Design review of the part built by this model. Coordinates are the model's own, in mm. Face numbers are marked on the shaded views. A direction names the side the tool comes from. Round coordinates to 2 decimals unless told otherwise and drop trailing zeros. Order: outer loops, then holes, each group sorted by start corner. A loop starts at its lowest first (then second) coordinate and runs counter-clockwise, first axis right, second up. Notation, with made-up numbers: (57.5, 14.25) - (84.5, 14.25) arc R29 ccw to (84.5, 45.25) - close; hole circle Ø3 at (15.5, -11). An arc over 180 degrees is marked (long way). Write item = value, one per line.
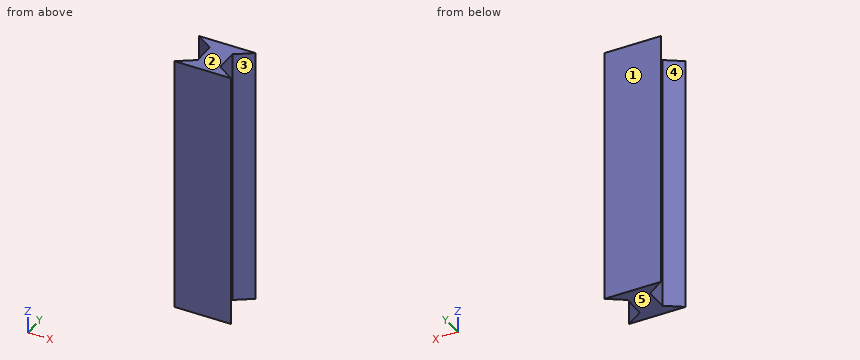
Autodesk Fusion 360 part; units mm, degrees
sketch "Sketch1" plane through (0, 0, 0) normal (0, 0, 1) x (1, 0, 0)
  line L0 (125, 0) -> (125, 1)
  line L1 (127, 0) -> (127, 1)
  line L2 (125, 0) -> (127, 0)
  line L3 (126, 0) -> (126, 2) construction
  line L4 (123.5, 2) -> (128.5, 2)
  line L5 (123.5, 2) -> (125, 1)
  line L6 (127, 1) -> (128.5, 2)
  line L7 (125, 0) -> (125, -1)
  line L8 (123.5, -2) -> (125, -1)
  line L9 (123.5, -2) -> (128.5, -2)
  line L10 (127, -1) -> (128.5, -2)
  line L11 (127, 0) -> (127, -1)
  line L12 (125, 0) -> (127, 0)
  dimension "d759" = 1
  dimension "d760" = 1
  dimension "d761" = 2
  dimension "d763" = 2
  dimension "d764" = 5
extrude "Extrude1" add sketch "Sketch1" along normal blind 23
Item 1: Take a section at D-D, the plane y = -1.2. State the section outline as (x, z) points, and give its area (3 significant figures).
Data:
outline = (124.7, 0) - (127.3, 0) - (127.3, 23) - (124.7, 23) - close
area = 59.8 mm2
Item 2: Take a section at C-C, the plane y = 0.45. State the section outline as (x, z) points, and give its area (3 significant figures).
Data:
outline = (125, 0) - (127, 0) - (127, 23) - (125, 23) - close
area = 46.0 mm2
Item 3: Take a section at B-B, the plane x = 124.75. State the section outline as (y, z) points.
Data:
outline = (-2, 0) - (-1.17, 0) - (-1.17, 23) - (-2, 23) - close; (1.17, 0) - (2, 0) - (2, 23) - (1.17, 23) - close
Item 4: For line 1 along X through (y, z) = (-0.4, 8.5); line 2 along Y through (x, z) = (127.95, 15.5); line 3 along Y through (x, z) = (123.9, 10), list the stretches that pass through material, from the lowest coordinate up. Write a range as [from, to].
Data:
line_1 = [125, 127]
line_2 = [-2, -1.63], [1.63, 2]
line_3 = [-2, -1.73], [1.73, 2]
Item 5: Insertion check: P1, Ø1.5, axis at y = 0, z = 14, coming from the -X side; P2, Ø0.6, axis at y = -0.5, z = 16, coming from the +X side. Each pin has a flat end and moves straight along its axis. Give the tip position at first contact, or say it passes through.
Data:
P1 = 125
P2 = 127
Item 6: For the marked faces 4 and 5, list the 3-axis set-ups (+Z, -Z, +X, -X, +Y, -Y) from which the entire face can be reached by the end or side of a thin tool; tool diameter is ignored.
Data:
face_4 = +Z, -Z, -X
face_5 = -Z, +X, -X, +Y, -Y
Item 7: The part is to be moulded in two halves that separate along Y. For the marked faces 1, 2 and 3, say which applies: +Y half, -Y half, draft (parallel to the pull), parting line (faces both ways), or undercut.
Data:
face_1 = +Y half
face_2 = draft
face_3 = undercut
Item 8: Take a section at A-A, the plane z = 18. State the section outline as (x, y) points, and give its area (3 significant figures).
Data:
outline = (123.5, -2) - (128.5, -2) - (127, -1) - (127, 1) - (128.5, 2) - (123.5, 2) - (125, 1) - (125, -1) - close
area = 11.0 mm2
